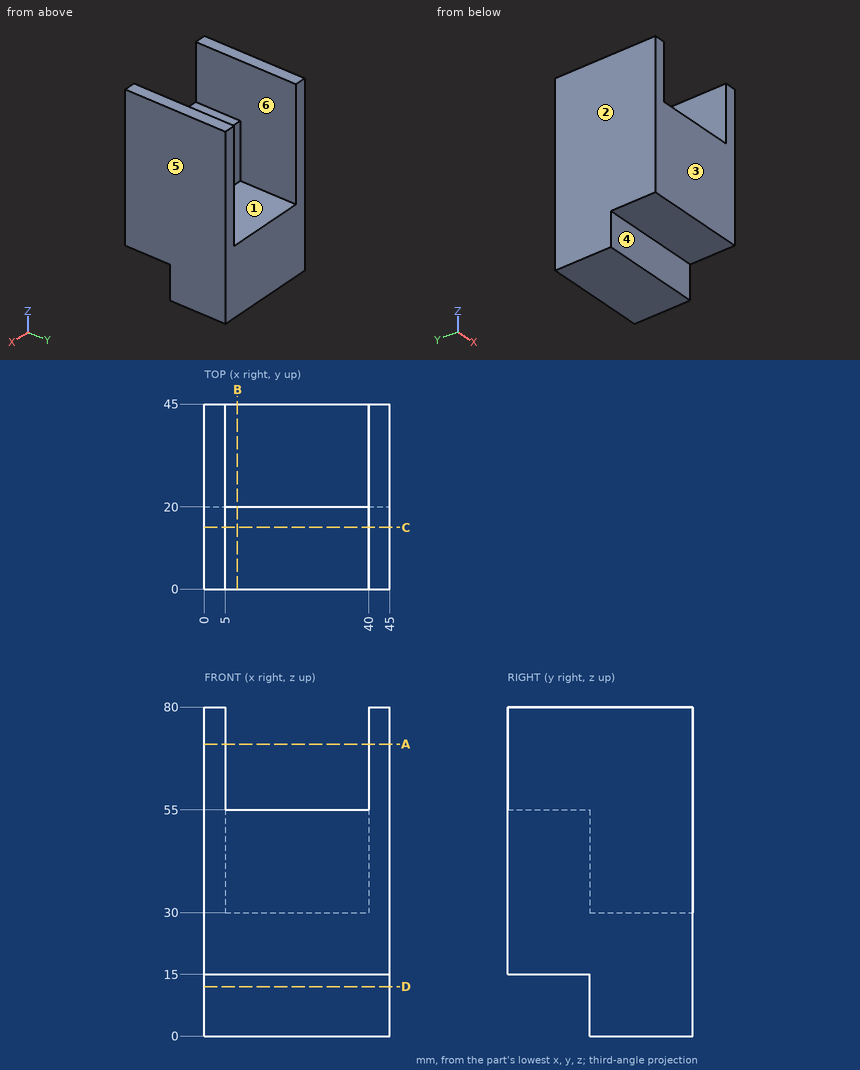
Design review of the part shown in the three views and the two pictorial views. Dimensions are in mm from the part's minimum x, y and z. A direction names the side the tool comes from. Give positions to 0.01 mm unless a question says otherwise; leave off trailing zeros. Loops run counter-clockwise (first coordinate to the right, second up) from the corner with the lowest first, then second, coordinate; pieces in that order, holes last. Notation, with made-up numbers: M -3,22 L 54,22 A10 cw 54,29 Z; hole C 14.5,-26 d1. An arc over 180 degrees is marked long. Answer as a JSON object with one key per item and string values. Group by question number.
Q1. For probe 1 along X at (y, z) = (14.5, 74); probe 2 along Z at (x, y) = (13.5, 32); probe 3 along Z at (x, y) = (41.5, 12), list the stretches that pass through material, from the lowest coordinate up. Write a range as [from, to].
Q2. Add section D-D on z = 12. Give the boundary of the cut face in (x, y), and give its area (4 significant figures).
Q3. Add section A-A on z = 71. Give the boundary of the cut face in (x, y), and give its area (3 significant figures).
Q4. Add section B-B on x = 8. Give the boundary of the cut face in (y, z).
Q5. Insertion check: P1, Ø12.5, axis at x = 15, z = 42, coming from the +Y side; P2, Ø12, axis at x = 28, y = 12, coming from the +Z side; P3, Ø6, axis at x = 22, y = 8.5, coming from the -Z side. Each pin has a flat end and moves straight along its axis. Give the tip position at first contact, or say it passes through.
Q6. Mouldability with a two-part tool opening along X and no side actions: class the marked faces 1, 2 and 3 as +X half, -X half, draft (parallel to the pull), parting line (faces both ways), or undercut.
Q7. Add section C-C on y = 15. Give the boundary of the cut face in (x, z), and give its area (3 significant figures).
Q8. Tool access review of the marked faces 4, 5 and 6: name each direction out of +Z, -Z, +X, -X, +Y, -Y from which nothing blocks a thin tool from reaching the whole face with its end or side.
Checked values:
{
 "1": {"probe 1": "[0, 5], [40, 45]", "probe 2": "[0, 30]", "probe 3": "[15, 80]"},
 "2": {"outline": "M 0,20 L 45,20 L 45,45 L 0,45 Z", "area": "1,125 mm²"},
 "3": {"outline": "M 0,0 L 5,0 L 5,45 L 0,45 Z; M 40,0 L 45,0 L 45,45 L 40,45 Z", "area": "450 mm²"},
 "4": {"outline": "M 0,15 L 20,15 L 20,0 L 45,0 L 45,30 L 20,30 L 20,55 L 0,55 Z"},
 "5": {"P1": "y = 20", "P2": "z = 55", "P3": "z = 15"},
 "6": {"face 1": "undercut", "face 2": "-X half", "face 3": "draft"},
 "7": {"outline": "M 0,15 L 45,15 L 45,80 L 40,80 L 40,55 L 5,55 L 5,80 L 0,80 Z", "area": "2,050 mm²"},
 "8": {"face 4": "-Z, +X, -X, -Y", "face 5": "+Z, -Z, +X, +Y, -Y", "face 6": "+Z, +Y"}
}
